Autodesk Inventor part; units mm, degrees
ref_plane "YZ Plane" through (0, 0, 0) normal (1, 0, 0) x (0, 1, 0)
ref_plane "XZ Plane" through (0, 0, 0) normal (0, 1, 0) x (-1, 0, 0)
ref_plane "XY Plane" through (0, 0, 0) normal (0, 0, 1) x (1, 0, 0)
sketch "Эскиз1" plane through (0, 0, 0) normal (0, 0, 1) x (1, 0, 0)
  circle A0 centre (142, -81.5) radius 3.75 construction
  circle A1 centre (142, -103.5) radius 3.75 construction
  circle A2 centre (142, -81.5) radius 1.75
  circle A3 centre (142, -103.5) radius 1.75
  line L0 (138, -77.5) -> (152, -77.5)
  line L1 (152, -77.5) -> (152, -107.5)
  line L2 (152, -107.5) -> (138, -107.5)
  line L3 (138, -107.5) -> (138, -77.5)
  line L4 (152, -77.5) -> (149, -77.5)
  line L5 (149, -77.5) -> (149, -107.5)
  line L6 (149, -107.5) -> (152, -107.5)
  line L7 (152, -107.5) -> (152, -77.5)
  point P0 (0, 0)
  dimension "d0" = 3.5
  dimension "d1" = 3.5
  dimension "d2" = 4
  dimension "d3" = 10
  dimension "d4" = 4
  dimension "d5" = 4
  dimension "d6" = 3
extrude "Выдавливание1" add sketch "Эскиз1" along normal blind 3
extrude "Выдавливание2" add sketch "Эскиз1" along normal blind 20 contours L0 L1 L2 L5
sketch "Эскиз2" plane through (149, -107.5, 3) normal (-1, 0, 0) x (0, 0, 1)
  circle A0 centre (7, 21) radius 2
  circle A1 centre (7, 9) radius 2
  line L0 (0, 30) -> (17, 30)
  line L1 (0, 0) -> (17, 0)
  line L2 (17, 30) -> (17, 0)
  point P0 (-3, 107.5)
  dimension "d11" = 4
  dimension "d12" = 4
  dimension "d13" = 12
  dimension "d14" = 9
  dimension "d16" = 10
  dimension "d17" = 10
extrude "Выдавливание3" cut sketch "Эскиз2" against normal blind 10
fillet "Сопряжение1" radius 5 4 edges at (150.5, -77.5, 20) (150.5, -107.5, 20) (138, -77.5, 1.5) (138, -107.5, 1.5)
properties part number "креление кабельканала"
CAD build for the part. Positions are in the model's coordinates, mm. A direction names the side the tool comes from. Round coordinates to 2 decimals unless told otherwise and drop trailing zeros. Write each loop counter-clockwise with the first axis right and the second up, starting at its lowest first coordinate (ties: lowest second). Pieces come first, ordered by that corner, then holes. Notation, with made-up numbers: (55, 36) - (102, 36) arc R20 cw to (102, 72) - close; hole circle Ø9 at (-4, 58). An arc over 180 degrees is marked (long way). Return JSON: item names as keys, results as strings. Group by question number.
Item 1: 3-axis set-ups, long thin cutter, end or side, ignore diameter. For faces 5 (the face through (143.669, -82.026, 1.479)), 6 (the face through (143, -92, 3)): which of +Z, -Z, +X, -X, +Y, -Y reach the whole face in a straight line?
Item 2: Probe probe 1 along Y at (x, z) = (150.5, 10); probe 2 along Y at (x, z) = (142, 1.05); probe 3 along X at (y, z) = (-82.5, 12.25). List the from-to ranges inside material, lowest first.
Item 3: Mould opens along Z. For faces 1 (the face through (150.48, -106.07, 18.5)), 2 (the face through (150.479, -96.517, 9.74)), 3 (the face through (150.479, -84.517, 9.74)), 4 (the face through (149, -92, 11)) say: +Z half, -Z half, draft (parallel to the pull), parting line (faces both ways), or undercut.
Item 4: Band-saw the part on A-A on z = 10. List the corners of the cut face in (x, y).
Item 5: Band-saw the part on D-D on z = 2. List the corners of the cut face in (x, y).
Item 6: Band-saw the part on B-B on y = -98.5. List the corners of the cut face in (x, z), plus the area to 3 significant figures.
Item 7: Flat gauge pins, fed straight in: pin 1 Ø1.5 at (x, y) = (140.5, -81) entering from -Z; pin 2 Ø2 at (y, z) = (-96.5, 8.5) entering from -X. Where does each tip first touch, or does it go through?
Item 8: Band-saw the part on C-C on x = 142. List the corners of the cut face in (y, z).
Resolved:
{
 "1": {"face 5": "+Z, -Z", "face 6": "+Z, -X, +Y, -Y"},
 "2": {"probe 1": "y = -107.5 to -100.5, -96.5 to -88.5, -84.5 to -77.5", "probe 2": "y = -107.4 to -105.25, -101.75 to -83.25, -79.75 to -77.6", "probe 3": "x = 149 to 152"},
 "3": {"face 1": "+Z half", "face 2": "undercut", "face 3": "undercut", "face 4": "draft"},
 "4": {"outline": "(149, -107.5) - (152, -107.5) - (152, -100.5) - (149, -100.5) - close; (149, -96.5) - (152, -96.5) - (152, -88.5) - (149, -88.5) - close; (149, -84.5) - (152, -84.5) - (152, -77.5) - (149, -77.5) - close"},
 "5": {"outline": "(138, -102.5) arc R5 ccw to (143, -107.5) - (152, -107.5) - (152, -77.5) - (143, -77.5) arc R5 ccw to (138, -82.5) - close; hole circle Ø3.5 at (142, -103.5); hole circle Ø3.5 at (142, -81.5)"},
 "6": {"outline": "(138, 0) - (152, 0) - (152, 8) - (149, 8) - (149, 3) - (138, 3) - close; (149, 12) - (152, 12) - (152, 20) - (149, 20) - close", "area": "81.0 mm²"},
 "7": {"pin 1": "stops at z = 0", "pin 2": "stops at x = 149"},
 "8": {"outline": "(-107.4, 0) - (-105.25, 0) - (-105.25, 3) - (-107.4, 3) - close; (-101.75, 0) - (-83.25, 0) - (-83.25, 3) - (-101.75, 3) - close; (-79.75, 0) - (-77.6, 0) - (-77.6, 3) - (-79.75, 3) - close"}
}
